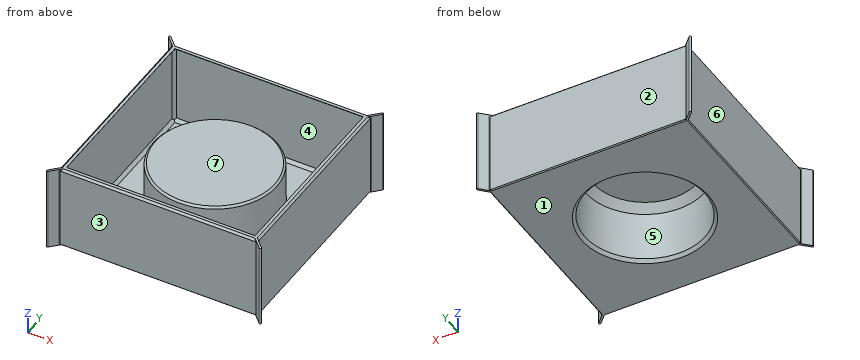
```python
from build123d import *

# Parameters (mm, degrees)
F0_W             = 80
F0_H             = 80
F1_DEPTH         = 34
F2_T             = -0.8
F3_R             = 25
F4_DEPTH         = 24
F4_TAPER         = 0.5
F5_T1_DEPTH      = 78.4
F5_T3_DEPTH      = 78.4
F6_W             = 80
F6_H             = 80
F6_W_2           = 76
F6_H_2           = 76
F7_DEPTH         = 0.05
F8_SIZE          = 1.19999
F11_DEPTH        = 34.05
F11_COPIES_COUNT = 4
F14_SIZE         = 3
F16_SIZE         = 0.4
F17_SIZE         = 0.8


# Not quite as in the source:
# - a fillet or chamfer that OpenCascade refuses, or shapes differently, is made with other operations: its cross-section is extruded or revolved along the edge and cut away or added
# - a fillet or chamfer is up to 0.001 mm smaller than in the source, because OpenCascade refuses the exact size
# - a pattern or mirror of a feature is missing from the dataset's text; its kind, count and spacing are read off the source's solid


with BuildPart() as f1:
    # F0 (on Top) → F1 (new body)
    with BuildSketch(Plane.XY):
        Rectangle(F0_W, F0_H)
    extrude(amount=F1_DEPTH)

    # F2
    f2_openings = [f1.faces().sort_by_distance(p)[0] for p in [
        (0, 0, 34),
    ]]
    offset(amount=F2_T, openings=f2_openings)

    # F3 (on face) → F4 (join)
    with BuildSketch(Plane.XY.offset(0.8)):
        Circle(F3_R)
    extrude(amount=F4_DEPTH, taper=F4_TAPER)

    # F5: chamfer of 1.2 on 5 edges, made by hand

    # F5_s2 → F5_t1 (join)
    with BuildSketch(Plane.XZ.offset(-39.2)):
        Polygon((-39.2, 2), (-38, 0.8), (-39.2, 0.8), align=None)
        Polygon((39.2, 2), (38, 0.8), (39.2, 0.8), align=None)
    extrude(amount=F5_T1_DEPTH)

    # F5_s4 → F5_t3 (join)
    with BuildSketch(Plane.YZ.offset(-39.2)):
        Polygon((-39.2, 2), (-38, 0.8), (-39.2, 0.8), align=None)
        Polygon((39.2, 2), (38, 0.8), (39.2, 0.8), align=None)
    extrude(amount=F5_T3_DEPTH)

    # F5_s5 → F5_t6 (revolve)
    with BuildSketch(Plane.XZ):
        Polygon((26.1895734527, 0.8), (24.989619145, 1.9895281574), (25, 0.8), align=None)
    revolve(axis=Axis((0, 0, 0.8), (0, 0, -1)))

    # F6 (on face) → F7 (join)
    with BuildSketch(Plane.XY.offset(34)):
        Rectangle(F6_W, F6_H)
        Rectangle(F6_W_2, F6_H_2, mode=Mode.SUBTRACT)
    extrude(amount=F7_DEPTH)

    # F8 (size 1.2 in the source; OpenCascade refuses exactly that, so slightly less here)
    f8_edges = [f1.edges().sort_by_distance(p)[0] for p in [
        (0, -39.2, 34),
        (-39.2, 0, 34),
        (-39.2, -39.2, 18),
        (-39.2, 39.2, 18),
        (0, 39.2, 34),
        (39.2, 0, 34),
        (39.2, 39.2, 18),
        (39.2, -39.2, 18),
    ]]
    chamfer(f8_edges, length=F8_SIZE)

    # F9: chamfer of 0.8 on 1 edges, made by hand

    # F9_s1 → F9_t2 (revolve, cut)
    with BuildSketch(Plane.XZ):
        Polygon((24.7975364014, 24.0000304615), (23.990555173, 24.8), (24.790555173, 24.8), align=None)
    revolve(axis=Axis((0, 0, 24.8), (0, 0, -1)), mode=Mode.SUBTRACT)

    # F10 (on face) → F11 (join, through all)
    with BuildSketch(Plane(origin=(0, 0, 0), x_dir=(1, 0, 0), z_dir=(0, 0, -1))):
        with BuildLine():
            Line((-39.1612012219, 39.7268866468), (-39.7171572875, 40.2828427125))
            ThreePointArc((-39.7171572875, 40.2828427125), (-39.7171572875, 39.7171572875), (-40.2828427125, 39.7171572875))
            Line((-40.2828427125, 39.7171572875), (-39.7268866468, 39.1612012219))
            Line((-39.7268866468, 39.1612012219), (-39.1612012219, 39.7268866468))
        make_face()
        with BuildLine():
            ThreePointArc((-40.2828427125, 39.7171572875), (-39.7171572875, 39.7171572875), (-39.7171572875, 40.2828427125))
            Line((-39.7171572875, 40.2828427125), (-42.5455844123, 43.1112698372))
            ThreePointArc((-42.5455844123, 43.1112698372), (-43.1112698372, 43.1112698372), (-43.1112698372, 42.5455844123))
            Line((-43.1112698372, 42.5455844123), (-40.2828427125, 39.7171572875))
        make_face()
    f11 = extrude(amount=-F11_DEPTH)

    # F11_copies: F11 ×4 about axis
    f11_copies_axis = Axis((0, 0, 0), (0, 0, 1))
    for i in range(1, F11_COPIES_COUNT):
        add(f11.rotate(f11_copies_axis, i * 360 / F11_COPIES_COUNT))

    # F12 (on Front) → F13 (revolve, cut)
    with BuildSketch(Plane.XZ):
        Polygon((-23.9975059387, 24.0000304615), (-24.2264749318, -2.2372173829), (0, -2.2372173829), (0, 24.0000304615), align=None)
    revolve(axis=Axis((0, 0, 10.8814065393), (0, 0, 1)), mode=Mode.SUBTRACT)

    # F14
    f14_edges = [f1.edges().sort_by_distance(p)[0] for p in [
        (23.997506, 0, 24.00003),
    ]]
    chamfer(f14_edges, length=F14_SIZE)

    # F15: chamfer of 1.2 on 1 edges, made by hand

    # F15_s1 → F15_t2 (revolve, cut)
    with BuildSketch(Plane.XZ):
        Polygon((-24.1964791889, 1.1999543077), (-25.4069510315, 0), (-24.2069510315, 0), align=None)
    revolve(axis=Axis((0, 0, 0), (0, 0, -1)), mode=Mode.SUBTRACT)

    # F16
    f16_edges = [f1.edges().sort_by_distance(p)[0] for p in [
        (0, -40, 0),
        (-40, 0, 0),
        (40, 0, 0),
        (0, 40, 0),
    ]]
    chamfer(f16_edges, length=F16_SIZE)

    # F17
    f17_edges = [f1.edges().sort_by_distance(p)[0] for p in [
        (0, -40, 34.05),
        (40, 0, 34.05),
        (0, 40, 34.05),
        (-40, 0, 34.05),
    ]]
    chamfer(f17_edges, length=F17_SIZE)


solid = f1.part
```
Input: part model. Units: mm. Frame: model coordinates. Face numbers are marked on the shaded views. A direction names the side the tool comes from. Coordinates: 2 decimals unless noted, no trailing zeros. Loops run counter-clockwise (first coordinate to the right, second up) from the corner with the lowest first, then second, coordinate; pieces in that order, holes last.
Q1. Mould query, pull axis Y, two halves, no side actions, for the marked faces 1, 2, 3 and 4. Classes: +Y half, -Y half, draft (parallel to the pull), parting line (faces both ways), or undercut.
Results are:
face 1: draft
face 2: +Y half
face 3: -Y half
face 4: undercut
Q2. Line query: line 1 along Y through (x, z) = (32, 16.5); line 2 along X through (y, z) = (6.5, 5). Output: solid intervals per line, ascending.
Results are:
line 1: y = -40 to -39.2, 39.2 to 40
line 2: x = -40 to -39.2, -24.1 to -23.27, 23.27 to 24.1, 39.2 to 40
Q3. Section A-A, the plane z = 26. Return the cut outline in (x, y), and give its area (3 significant figures).
Results are:
outline: (-43.11, -42.55) arc R0.4 ccw to (-42.55, -43.11) - (-39.43, -40) - (39.43, -40) - (42.55, -43.11) arc R0.4 ccw to (43.11, -42.55) - (40, -39.43) - (40, 39.43) - (43.11, 42.55) arc R0.4 ccw to (42.55, 43.11) - (39.43, 40) - (-39.43, 40) - (-42.55, 43.11) arc R0.4 ccw to (-43.11, 42.55) - (-40, 39.43) - (-40, -39.43) - close; hole (-39.2, -38) - (-38, -39.2) - (38, -39.2) - (39.2, -38) - (39.2, 38) - (38, 39.2) - (-38, 39.2) - (-39.2, 38) - close
area: 271 mm2
Q4. Set-up query: the marked faces 5, 6 and 7. Return all of +Z, -Z, +X, -X, +Y, -Y with unobstructed straight access to the full face (end or side cutting, diameter ignored); none if empty.
Results are:
face 5: -Z
face 6: +Z, -Z, -X
face 7: +Z
Q5. Contact query for flat-ended pins moving along their axis: pin 1 (9 mm diameter, centred on x = 14, z = 14.5, fed in from +Y); pin 2 (10 mm diameter, centred on y = 8, z = 26.5, fed in from +X); pin 3 (3 mm diameter, centred on x = -3, y = 7, fed in from -Z). Output: stop coordinate, or through.
Results are:
pin 1: stops at y = 40
pin 2: stops at x = 40
pin 3: stops at z = 24
